Verification items for the finished model (mm, model axes). Coordinates: 2 decimals unless noted, no trailing zeros. Order: outer loops, then holes, each group sorted by start corner. A loop starts at its lowest first (then second) coordinate and runs counter-clockwise, first axis right, second up. Notation, with made-up numbers: (-8, 30) -> (31, 30) arc R15 cw to (31, 47) -> close; hole circle Ø4 at (69, -17.5). An arc over 180 degrees is marked (long way). Write item = value, one per line. Start each with the question number.
Autodesk Inventor part; units mm, degrees
ref_plane "YZ Plane" through (0, 0, 0) normal (1, 0, 0) x (0, 1, 0)
ref_plane "XZ Plane" through (0, 0, 0) normal (0, 1, 0) x (-1, 0, 0)
ref_plane "XY Plane" through (0, 0, 0) normal (0, 0, 1) x (1, 0, 0)
ref_plane "Work Plane1" through (-0.0049, -0.13, 0) normal (0, 0, 1) x (1, 0, 0)
sketch "Sketch1" plane through (-0.0049, -0.13, 0) normal (0, 0, 1) x (1, 0, 0)
  line L0 (0.0049, 0.13) -> (-63.4951, 0.13)
  line L1 (-63.4951, 0.13) -> (-63.4951, -482.47)
  line L2 (-63.4951, -482.47) -> (0.0049, -482.47)
  line L3 (0.0049, -482.47) -> (0.0049, 0.13)
  line L4 (-63.4951, -482.47) -> (114.3049, -482.47)
  line L5 (-63.4951, -482.47) -> (114.3049, -482.47) construction
  line L6 (-63.4951, -482.47) -> (63.5049, -482.47)
  line L7 (63.5049, -482.47) -> (63.5049, -406.27)
  line L8 (63.5049, -406.27) -> (-63.4951, -406.27)
  line L9 (-63.4951, -406.27) -> (-63.4951, -482.47)
  line L10 (-63.4951, -482.47) -> (-63.4951, -914.27)
  line L11 (-63.4951, -482.47) -> (368.3049, -482.47) construction
  line L12 (-63.4951, -914.27) -> (114.3049, -914.27)
  line L13 (114.3049, -914.27) -> (114.3049, -482.47)
  line L14 (-63.4951, -406.27) -> (-63.4951, -393.57)
  line L15 (-63.4951, -406.27) -> (-50.7951, -406.27) construction
  line L16 (-63.4951, -393.57) -> (-317.4951, -393.57)
  line L17 (-63.4951, -393.57) -> (190.5049, -393.57) construction
  line L18 (-63.4951, -393.57) -> (-317.4951, -393.57)
  line L19 (-317.4951, -393.57) -> (-317.4951, -914.27)
  line L20 (-317.4951, -914.27) -> (-63.4951, -914.27)
  line L21 (-63.4951, -914.27) -> (-63.4951, -393.57)
  line L22 (-63.4951, -393.57) -> (-177.7951, -393.57)
  line L23 (-177.7951, -393.57) -> (114.3049, -685.67)
  line L24 (114.3049, -685.67) -> (114.3049, -914.27)
  line L25 (-177.7951, -393.57) -> (114.3049, -685.6537)
  line L26 (-177.7951, -393.57) -> (-177.7951, -990.597)
  line L27 (-177.7951, -393.57) -> (419.2319, -393.57) construction
  line L28 (-177.7951, -990.597) -> (-65.9571, -791.2225)
  line L29 (-177.7951, -990.597) -> (50.8049, -990.597) construction
  line L30 (-65.9571, -791.2225) -> (-177.7951, -393.57)
  line L31 (-134.9799, -914.27) -> (-157.1327, -901.8436)
  line L32 (-134.9799, -914.27) -> (-109.5799, -914.27) construction
  line L33 (-157.1327, -901.8436) -> (-95.0804, -791.2225)
  line L34 (-75.3464, -757.8376) -> (-99.7978, -764.7145)
  line L35 (-95.0804, -791.2225) -> (-93.2568, -787.9716)
  line L36 (-93.2568, -787.9716) -> (-204.1924, -393.57)
  line L37 (-93.2568, -787.9716) -> (316.4496, -787.9716) construction
  line L38 (-190.4951, -393.57) -> (-193.9339, -381.3444)
  line L39 (-190.4951, -393.57) -> (-177.7951, -393.57) construction
  line L40 (-204.1924, -393.57) -> (-207.1501, -383.0548)
  line L41 (-193.9339, -381.3444) -> (-206.6269, -384.9147)
  line L42 (-206.6269, -384.9147) -> (-176.4218, -376.4187)
  line L43 (-177.7951, -393.57) -> (-182.165, -378.0341)
  line L44 (-182.165, -378.0341) -> (-206.6269, -384.9147)
  line L45 (-206.6269, -384.9147) -> (-93.2568, -787.9716)
  line L46 (-190.4951, -393.57) -> (-177.7951, -393.57)
  line L47 (-177.7951, -393.57) -> (-182.165, -378.0341)
  line L48 (-182.165, -378.0341) -> (-193.9339, -381.3444)
  line L49 (-193.9339, -381.3444) -> (-190.4951, -393.57)
  dimension "d0" = 63.5
  dimension "d1" = 482.6
  dimension "d2" = 177.8
  dimension "d3" = 0
  dimension "d4" = 127
  dimension "d5" = 76.2
  dimension "d6" = 431.8
  dimension "d7" = 90
  dimension "d8" = 12.7
  dimension "d9" = 90
  dimension "d10" = 254
  dimension "d11" = 180
  dimension "d12" = 254
  dimension "d13" = 520.7
  dimension "d14" = 114.3
  dimension "d15" = 45
  dimension "d16" = 413.0802
  dimension "d17" = 597.027
  dimension "d18" = 90
  dimension "d19" = 228.6
  dimension "d20" = 60.71
  dimension "d21" = 25.4
  dimension "d22" = 150.71
  dimension "d23" = 25.4
  dimension "d25" = 105.71
  dimension "d26" = 12.7
  dimension "d27" = 105.71
extrude "Extrusion1" add sketch "Sketch1" along normal blind 25.4 contours L26 L36 L16 | L30 L34 L36 L26 | L16 L38 L42 L43 | L16 L40 L41 L38 | L30 L28 L31 L33 L35 L36 L34
sketch "Sketch2" plane through (-0.0049, -0.13, 25.4) normal (0, 0, 1) x (1, 0, 0)
  line L0 (-182.165, -378.0341) -> (-206.6269, -384.9147)
  line L1 (-206.6269, -384.9147) -> (-182.165, -378.0341)
  line L2 (-182.165, -378.0341) -> (-194.396, -381.4744)
  line L3 (-194.396, -381.4744) -> (-190.9572, -393.7)
  circle A0 centre (-190.9572, -393.7) radius 3.175
  point P0 (0.0049, 0.13)
  dimension "d30" = 12.7
  dimension "d31" = 6.35
extrude "Extrusion2" cut sketch "Sketch2" against normal blind 25.4
properties part number "V-Arm"
Item 1: Gauge pin test, flat ends, axial feed: P1, Ø5.5, axis at x = -190.96, y = -393.83, coming from the +Z side; P2, Ø12, axis at y = -682, z = 17, coming from the -X side; P3, Ø1.5, axis at y = -839.5, z = 14, coming from the +X side; P4, Ø10, axis at y = -860, z = 15, coming from the -X side. Record the tip position at first contact, or that the pin passes through.
Item 2: Thickness scan on line 1 (X direction, y = -393.83, z = 13.25); line 2 (X direction, y = -821, z = 6); line 3 (X direction, y = -537.5, z = 11.25). Record the ranges inside material, lowest first.
Item 3: Section check B-B (y = -764). Record the boundary of the cut face in (x, z), then the cut area to 3 significant figures.
Item 4: Section check C-C (y = -825.5). Record the boundary of the cut face in (x, z), then the cut area to 3 significant figures.
Filled sheet:
q1.P1 = through
q1.P2 = -124.79
q1.P3 = -92.55
q1.P4 = -136.4
q2.line_1 = -204.16 to -194.14, -187.79 to -177.76
q2.line_2 = -111.72 to -82.59
q2.line_3 = -163.75 to -137.36
q3.outline = (-100.04, 0) -> (-73.65, 0) -> (-73.65, 25.4) -> (-100.04, 25.4) -> close
q3.area = 670 mm^2
q4.outline = (-114.24, 0) -> (-85.12, 0) -> (-85.12, 25.4) -> (-114.24, 25.4) -> close
q4.area = 740 mm^2
